Geometry: final body of the model. Coordinates: model frame, mm. A direction names the side the tool comes from. Round coordinates to 2 decimals unless told otherwise and drop trailing zeros. Write each loop counter-clockwise with the first axis right and the second up, starting at its lowest first coordinate (ties: lowest second). Pieces come first, ordered by that corner, then holes.
from build123d import *

# Parameters (mm, degrees)
F0_W     = 31.28859
F0_H     = 49.892618
F1_DEPTH = 25
F2_R     = 5.101278
F3_DEPTH = 25
F4_W     = 23.469856
F4_H     = 2.933731
F5_DEPTH = 25


with BuildPart() as f1:
    # F0 (on Top) → F1 (new body)
    with BuildSketch(Plane.XY):
        with BuildLine():
            ThreePointArc((14.692953, 24.100671), (-0.951342, 39.744966), (-16.595637, 24.100671))
            Line((-16.595637, 24.100671), (14.692953, 24.100671))
        make_face()
        with Locations((-0.951342, -0.845638)):
            Rectangle(F0_W, F0_H)
        with BuildLine():
            Line((14.692953, -25.791947), (-16.595637, -25.791947))
            ThreePointArc((-16.595637, -25.791947), (-0.951342, -41.436242), (14.692953, -25.791947))
        make_face()
    extrude(amount=F1_DEPTH)

    # F2 (on Top) → F3 (cut)
    with BuildSketch(Plane.XY):
        with Locations((0, 26.003355)):
            Circle(F2_R)
    extrude(amount=F3_DEPTH, mode=Mode.SUBTRACT)

    # F4 (on face) → F5 (cut)
    with BuildSketch(Plane(origin=(0, 0, 0), x_dir=(1, 0, 0), z_dir=(0, 0, -1))):
        with Locations((14.623049, -26.399825)):
            Rectangle(F4_W, F4_H)
    extrude(amount=-F5_DEPTH, mode=Mode.SUBTRACT)


solid = f1.part
1) Section A-A on y = 29. Output: boundary loops of the cut face in (x, z), plus the area to 3 significant figures.
2) Reachability of faces 1 (the flat face through (10, 24.933, 12)), 2 (the flat face through (-16.596, -1, 12)) from +Z, -Z, +X, -X, +Y, -Y: full face, straight path, thin tool, end or side. Return the list, or none.
3) Section B-B on x = 0. Output: boundary loops of the cut face in (y, z), plus the area to 3 significant figures.
4) Section C-C on z = 13.75. Output: boundary loops of the cut face in (x, y), plus the area to 3 significant figures.
5) Line query: probe 1 along Y at (x, z) = (3, 18.5); probe 2 along Y at (x, z) = (4, 14.75); probe 3 along X at (y, z) = (22, 8.25). Output: solid intervals per line, ascending.
6) Draft query along Y for faces 3 (the cylindrical face through (-2.533, 39.665, 12.325)), 4 (the flat face through (9, 27.867, 12)), 5 (the flat face through (14.693, -1, 12)). Return one class per face: pulls with the +Y half, pulls with the -Y half, needs draft (parallel to the pull), parting line crosses it, or undercut.
7) First-contact query: P1, Ø4, axis at y = 28.5, z = 10, coming from the +X side; P2, Ø1, axis at x = 2.5, z = 14.5, coming from the -Y side; P3, Ø1.5, axis at x = 7, z = 14, coming from the -Y side. Flat tips, straight axial feed; report the tip coordinate or a pass-through.
Filled in:
1. outline: (-15.81, 0) - (-4.13, 0) - (-4.13, 25) - (-15.81, 25) - close; (4.13, 0) - (13.91, 0) - (13.91, 25) - (4.13, 25) - close
1. area: 536 mm2
2. face 1: +Z, -Z, +X
2. face 2: +Z, -Z, -X, +Y, -Y
3. outline: (-41.41, 0) - (20.9, 0) - (20.9, 25) - (-41.41, 25) - close; (31.1, 0) - (39.72, 0) - (39.72, 25) - (31.1, 25) - close
3. area: 1,770 mm2
4. outline: (-16.6, -25.79) arc R15.64 ccw to (14.69, -25.79) - (14.69, 24.1) arc R15.64 ccw to (14.67, 24.93) - (4.99, 24.93) arc R5.1 cw (long way) to (4.75, 27.87) - (14.23, 27.87) arc R15.64 ccw to (-16.6, 24.1) - close
4. area: 2,220 mm2
5. probe 1: y = -40.93 to 21.88, 30.13 to 39.24
5. probe 2: y = -40.63 to 22.84, 29.17 to 38.94
5. probe 3: x = -16.6 to -3.16, 3.16 to 14.69
6. face 3: pulls with the +Y half
6. face 4: undercut
6. face 5: needs draft
7. P1: stops at x = 14.23
7. P2: stops at y = -41.16
7. P3: stops at y = -39.68
